Geometry: see drawing. Coordinates: mm, zero at the bounding-box minimum. Coordinates: 2 decimals unless noted, no trailing zeros. Order: outer loops, then holes, each group sorted by start corner. A loop starts at its lowest first (then second) coordinate and runs counter-clockwise, first axis right, second up.
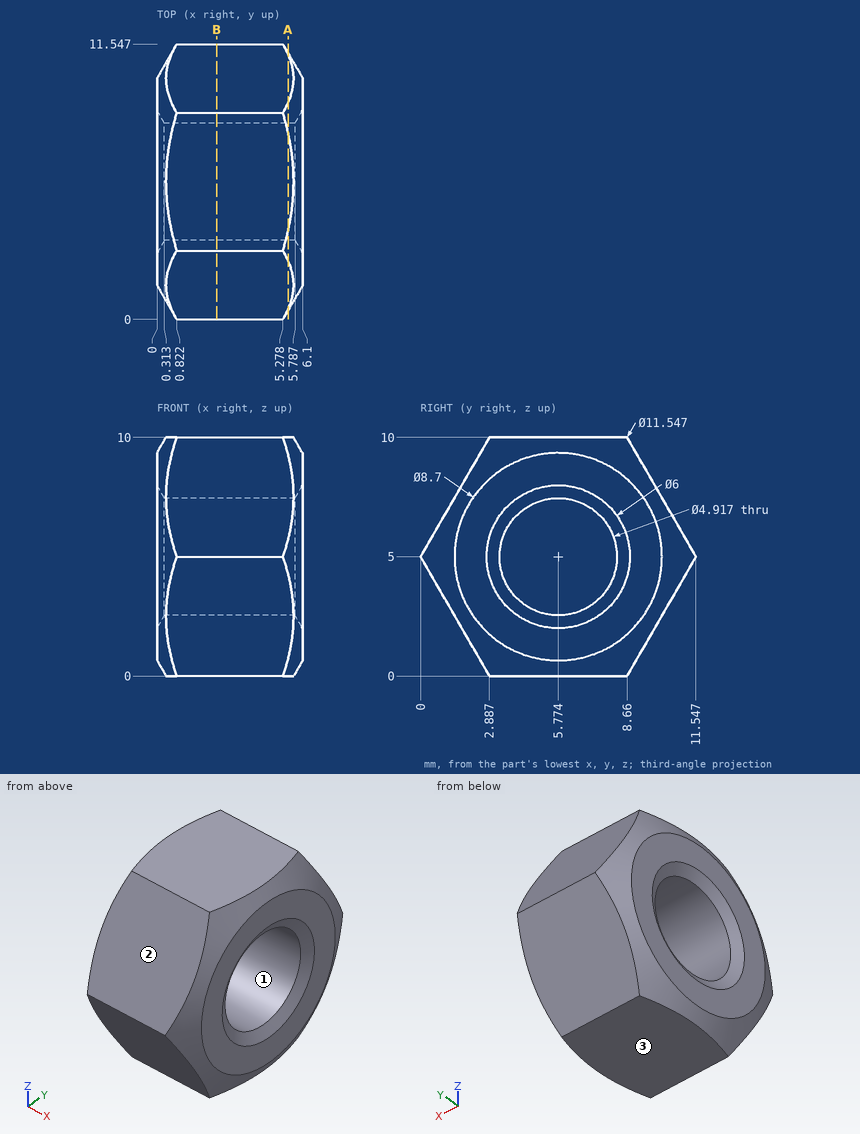
Item 1: Cut plane B-B on x = 2.5. Return loops of the section in (y, z).
Response values:
outline: (0, 5) - (2.89, 0) - (8.66, 0) - (11.55, 5) - (8.66, 10) - (2.89, 10) - close; hole circle Ø4.92 at (5.77, 5)
Item 2: Ray query, probe 1 along Z at (x, y) = (4.5, 5.75); probe 2 along Y at (x, z) = (4, 3.25) (1 decimal); probe 3 along Z at (x, y) = (0.75, 6.25). Return the intervals inside material, ascending.
Response values:
probe 1: z = 0 to 2.54, 7.46 to 10
probe 2: y = 1 to 4, 7.5 to 10.5
probe 3: z = 0 to 2.59, 7.41 to 10
Item 3: Draft query along Z for the marked faces 1, 2 and 3. Return one class per face: pulls with the +Z half, pulls with the -Z half, needs draft (parallel to the pull), parting line crosses it, or undercut.
Response values:
face 1: undercut
face 2: pulls with the +Z half
face 3: pulls with the -Z half
Item 4: Cut plane A-A on x = 5.5. Return loops of the section in (y, z) (1 decimal).
Response values:
outline: (0.4, 4.2) - (2.4, 0.8) arc R5.4 ccw to (3.8, 0) - (7.8, 0) arc R5.4 ccw to (9.1, 0.8) - (11.1, 4.2) arc R5.4 ccw to (11.1, 5.8) - (9.1, 9.2) arc R5.4 ccw to (7.8, 10) - (3.8, 10) arc R5.4 ccw to (2.4, 9.2) - (0.4, 5.8) arc R5.4 ccw to start; hole circle Ø4.9 at (5.8, 5)
